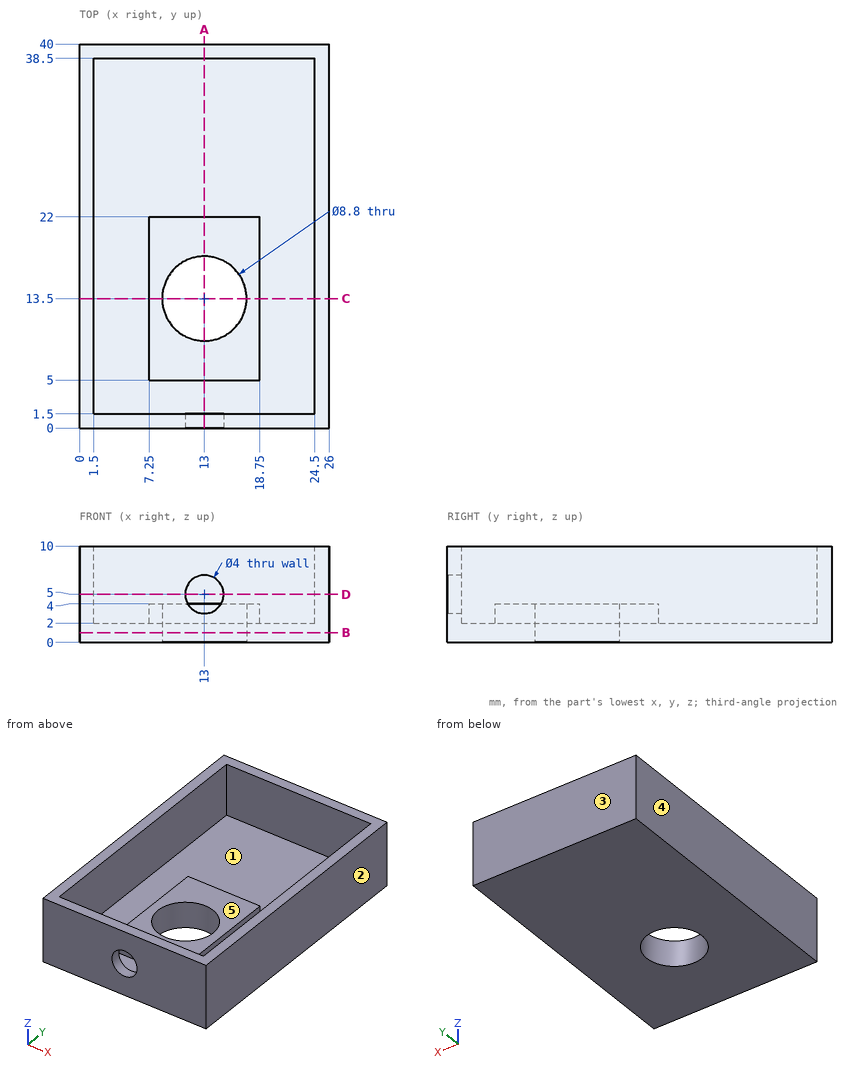
Drawing for the job (mm, zero at the part's lowest x, y, z). A direction names the side the tool comes from. Give positions to 0.01 mm unless a question says otherwise; leave off trailing zeros. Order: outer loops, then holes, each group sorted by start corner. A loop starts at its lowest first (then second) coordinate and runs counter-clockwise, first axis right, second up. Notation, with made-up numbers: M 86,63.25 L 131,63.25 A20 cw 131,78.25 Z; hole C 87,18.5 d7. An arc over 180 degrees is marked long. Put each result on its own line as item: value.
Item 1: Slice it at A-A, the plane x = 13. Write the cut outline in (y, z).
From the geometry:
outline: M 0,0 L 9.1,0 L 9.1,4 L 5,4 L 5,2 L 1.5,2 L 1.5,3 L 0,3 Z; M 0,7 L 1.5,7 L 1.5,10 L 0,10 Z; M 17.9,0 L 40,0 L 40,10 L 38.5,10 L 38.5,2 L 22,2 L 22,4 L 17.9,4 Z
Item 2: Slice it at B-B, the plane z = 1. Write the cut outline in (x, y), plus the area to 3 significant figures.
From the geometry:
outline: M 0,0 L 26,0 L 26,40 L 0,40 Z; hole C 13,13.5 d8.8
area: 979 mm2
Item 3: Flat gauge pins, fed straight in: pin 1 Ø3 at (x, z) = (13, 5) entering from -Y; pin 2 Ø3 at (x, y) = (17.5, 10.5) entering from +Z. Where does each tip first touch, or does it go through?
From the geometry:
pin 1: stops at y = 5
pin 2: stops at z = 4
Item 4: Two-plate mould, pull along Y, no slides. Class the marked faces 1, 2 and 3: +Y half, -Y half, draft (parallel to the pull), parting line (faces both ways), or undercut.
From the geometry:
face 1: undercut
face 2: draft
face 3: +Y half
Item 5: Slice it at C-C, the plane y = 13.5. Write the cut outline in (x, z), plus the area to 3 significant figures.
From the geometry:
outline: M 0,0 L 8.6,0 L 8.6,4 L 7.25,4 L 7.25,2 L 1.5,2 L 1.5,10 L 0,10 Z; M 17.4,0 L 26,0 L 26,10 L 24.5,10 L 24.5,2 L 18.75,2 L 18.75,4 L 17.4,4 Z
area: 63.8 mm2
Item 6: Slice it at D-D, the plane z = 5. Write the cut outline in (x, y).
From the geometry:
outline: M 0,0 L 11,0 L 11,1.5 L 1.5,1.5 L 1.5,38.5 L 24.5,38.5 L 24.5,1.5 L 15,1.5 L 15,0 L 26,0 L 26,40 L 0,40 Z
Item 7: Probe line 1 (Y direction, x = 13, z = 2.3); line 2 (Y direction, x = 5.5, z = 3.25); line 3 (X direction, y = 9, z = 4.5). List the from-to ranges inside material, lowest first. Write a range as [from, to].
From the geometry:
line 1: y = [0, 1.5], [5, 9.1], [17.9, 22], [38.5, 40]
line 2: y = [0, 1.5], [38.5, 40]
line 3: x = [0, 1.5], [24.5, 26]
Item 8: 3-axis set-ups, long thin cutter, end or side, ignore diameter. For the marked faces 4 and 5: which of +Z, -Z, +X, -X, +Y, -Y reach the whole face in a straight line?
From the geometry:
face 4: +Z, -Z, -X, +Y, -Y
face 5: +Z
